Verification items for the finished model (mm, model axes). A direction names the side the tool comes from. Give positions to 0.01 mm unless a question says otherwise; leave off trailing zeros. Order: outer loops, then holes, each group sorted by start corner. A loop starts at its lowest first (then second) coordinate and runs counter-clockwise, first axis right, second up.
Autodesk Inventor part; units mm, degrees
ref_plane "Work Plane1" through (-121.6053, -233.9347, 42.0294) normal (0, 0, -1) x (0, 1, 0)
ref_plane "YZ Plane" through (0, 0, 0) normal (1, 0, 0) x (0, 1, 0)
ref_plane "XZ Plane" through (0, 0, 0) normal (0, 1, 0) x (-1, 0, 0)
sketch "Sketch1" plane through (0, 0, 0) normal (0, 0, 1) x (1, 0, 0)
  line L0 (79.395, -155.8766) -> (79.395, 6.5)
  line L1 (-8.605, 6.5) -> (-8.605, -107.0766)
  line L2 (69.9453, -18.7158) -> (55.4353, -18.7158)
  line L3 (79.395, -18.7158) -> (79.395, -23.7158)
  line L4 (79.395, -23.7158) -> (71.895, -23.7158)
  line L5 (71.895, -23.7158) -> (71.895, -31.2158)
  line L6 (71.895, -31.2158) -> (79.395, -31.2158)
  line L7 (79.395, -31.2158) -> (79.395, -23.7158)
  point P0 (0, 0)
  dimension "d0" = 5
  dimension "d1" = 7.5
  dimension "d2" = 7.5
ref_plane "Work Plane1" through (-121.6053, -233.9347, 42.0294) normal (0, 0, -1) x (0, 1, 0)
extrude "Extrusion1" add sketch "Sketch1" along normal up to surface (42.0294 mm away)
sketch "Sketch2" plane through (71.895, -23.7158, 42.0294) normal (0, 0, 1) x (1, 0, 0)
  line L0 (7.5, 0) -> (0, 0)
  line L1 (0, 0) -> (15, 0)
  line L2 (15, 0) -> (15, -7.5)
  line L3 (15, -7.5) -> (0, -7.5)
  line L4 (0, -7.5) -> (0, 0)
  point P0 (-71.895, 23.7158)
  dimension "d5" = 15
extrude "Extrusion2" add sketch "Sketch2" against normal blind 3
fillet "Fillet1" radius 1 6 edges at (79.395, -23.7158, 19.5147) (71.895, -23.7158, 21.0147) (79.395, -31.2158, 19.5147) (71.895, -31.2158, 21.0147) (86.895, -23.7158, 40.5294) (86.895, -31.2158, 40.5294)
fillet "Fillet2" radius 1 5 edges at (86.6021, -30.9229, 39.0294) (78.895, -31.2158, 39.0294) (86.6021, -24.0087, 39.0294) (78.895, -23.7158, 39.0294) (86.895, -27.4658, 39.0294)
fillet "Fillet3" radius 1 1 edges at (79.395, -27.4658, 39.0294)
properties part number "TableLeg"
(1) Section check C-C, the plane x = 81. Enter the section's corners in (y, z).
Solved:
outline: (-31.22, 40.03) arc R1 ccw to (-30.22, 39.03) - (-24.72, 39.03) arc R1 ccw to (-23.72, 40.03) - (-23.72, 42.03) - (-31.22, 42.03) - close
(2) Scan lines: line 1 (X direction, y = -26, z = 35.5) (3 decimals); line 2 (Z direction, x = 84.75, y = -25). Record each from-to range of solid material in increasing order.
Solved:
line 1: x = 71.895 to 79.395
line 2: z = 39.03 to 42.03
(3) Section check B-B, the plane z = 12.5. Enter the section's corners in (x, y) (3 decimals), then the cut area to 3 significant figures.
Solved:
outline: (71.895, -30.216) arc R1 ccw to (72.895, -31.216) - (78.395, -31.216) arc R1 ccw to (79.395, -30.216) - (79.395, -24.716) arc R1 ccw to (78.395, -23.716) - (72.895, -23.716) arc R1 ccw to (71.895, -24.716) - close
area: 55.4 mm2
(4) Set-up check for faces 1 (the cylindrical face through (82.93, -24, 39.33)), 2 (the cylindrical face through (83, -30.9, 39.3)), 3 (the cylindrical face through (86.594, -24.001, 41.015)), 4 (the flat face through (75, -23.716, 21)), 5 (the flat face through (79.395, -28, 19)): record each of +Z, -Z, +X, -X, +Y, -Y from which the full face is reachable in a straight line by a thin tool's end or side.
Solved:
face 1: -Z, +X, +Y
face 2: -Z, +X, -Y
face 3: +Z, -Z, +X, +Y
face 4: +Z, -Z, +X, -X, +Y
face 5: -Z, +X, +Y, -Y
(5) Section check A-A, the plane y = -27.75. Enter the section's corners in (x, z) (3 decimals), then the cut area to 3 significant figures.
Solved:
outline: (71.895, 0) - (79.395, 0) - (79.395, 38.029) arc R1 cw to (80.395, 39.029) - (85.895, 39.029) arc R1 ccw to (86.895, 40.029) - (86.895, 42.029) - (71.895, 42.029) - close
area: 338 mm2
(6) Go/stop test with flat-tipped pins: pin 1 (4.5 mm diameter, centred on x = 84, y = -27.5, fed in from -Z); pin 2 (8 mm diameter, centred on x = 83, z = 21.5, fed in from -Y); pin 3 (3 mm diameter, centred on y = -28.5, z = 19.5, fed in from +X) (3 decimals); pin 4 (3 mm diameter, centred on x = 81, z = 26, fed in from +Y). Record where each tip stops, or that it passes through.
Solved:
pin 1: stops at z = 39.03
pin 2: stops at y = -31.01
pin 3: stops at x = 79.395
pin 4: passes through
